The model under review builds one solid part; all positions refer to its coordinate system, in mm. Face numbers are marked on the shaded views. A direction names the side the tool comes from. Round coordinates to 2 decimals unless told otherwise and drop trailing zeros. Order: outer loops, then holes, each group sorted by start corner. A loop starts at its lowest first (then second) coordinate and runs counter-clockwise, first axis right, second up.
1) Machinability: for the marked faces 1, 2, 3 and 4, which of the approach directions +Z, -Z, +X, -X, +Y, -Y give a long, thin tool a straight path to every point of the face, cutting with its end or side? Answer none if there is none.
2) Consider section A-A (y = -14.5). Give the boundary of the cut face in (x, z), then the cut area to 3 significant figures.
3) Consider section B-B (y = -29.5). Give the boundary of the cut face in (x, z), then the cut area to 3 significant figures.
4) Clearance check with flat-ended pins moving along their axes: P1, Ø1.5, axis at y = -12, z = 23.5, coming from the -X side; P2, Ø1.5, axis at x = -19, z = -19.5, coming from the -Y side; P3, Ø4, axis at x = -18.5, y = -9, coming from the +Z side; P4, Ø5, axis at x = -37, z = 37, coming from the -Y side. State where each tip first meets the part, or that it passes through.
5) Mouldability with a two-part tool opening along Z and no side actions: class the marked faces 5, 6 and 7 as pulls with the +Z half, pulls with the -Z half, needs draft (parallel to the pull), parting line crosses it, or undercut.
6) To check wall thickness, follow L1, parallel to Z at x = 37, y = -1; L2, parallel to Z at x = 0, y = -4.35; L3, parallel to Y at x = -34.5, z = -31.5. State the ranges of each line that lie inside material, in increasing order.
from build123d import *

# Parameters (mm, degrees)
F2_W     = 85
F2_H     = 85
F2_R     = 2.75
F3_DEPTH = 5
F4_SIZE  = 1.5
F5_R     = 15
F6_DEPTH = 2


with BuildPart() as f1:
    # F0 (on Right) → F1 (revolve)
    with BuildSketch(Plane.YZ):
        Polygon((-5, 0), (0, 0), (0, 42.5), (-32, 42.5), (-32, 37.7), (-17, 37.7), (-17, 21.2), (-5, 21.2), align=None)
    revolve(axis=Axis((0, -2.5, 0), (0, 1, 0)))

    # F2 (on Front) → F3 (join)
    with BuildSketch(Plane.XZ):
        Rectangle(F2_W, F2_H)
        with Locations((-37, -37)):
            Circle(F2_R, mode=Mode.SUBTRACT)
        with Locations((37, -37)):
            Circle(F2_R, mode=Mode.SUBTRACT)
        with Locations((-37, 37)):
            Circle(F2_R, mode=Mode.SUBTRACT)
        with Locations((37, 37)):
            Circle(F2_R, mode=Mode.SUBTRACT)
    extrude(amount=F3_DEPTH)

    # F4
    f4_edges = [f1.edges().sort_by_distance(p)[0] for p in [
        (0, -32, -37.7),
        (0, -17, -21.2),
        (42.5, -2.5, 42.5),
        (-42.5, -2.5, 42.5),
        (-42.5, -2.5, -42.5),
        (42.5, -2.5, -42.5),
    ]]
    chamfer(f4_edges, length=F4_SIZE)

    # F5 (on face) → F6 (cut)
    with BuildSketch(Plane.XZ.offset(5)):
        Circle(F5_R)
    extrude(amount=-F6_DEPTH, mode=Mode.SUBTRACT)


solid = f1.part
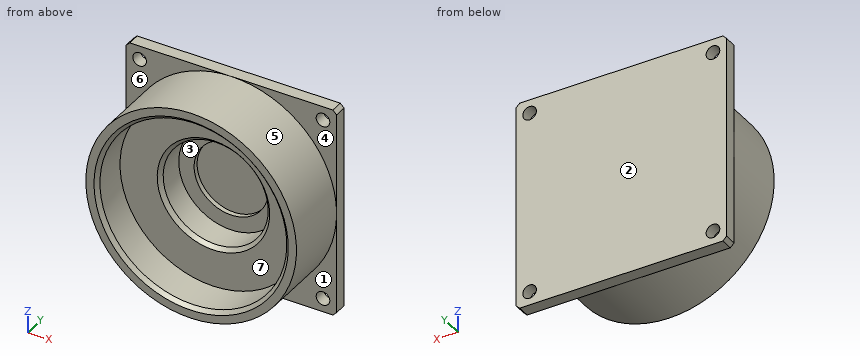
Answer below:
1. face 1: -Z, +X, -Y
1. face 2: +Z, -Z, +X, -X, +Y
1. face 3: -Y
1. face 4: +Z, +X, -Y
2. outline: circle Ø85 at (0, 0); hole circle Ø42.4 at (0, 0)
2. area: 4,260 mm2
3. outline: circle Ø85 at (0, 0); hole circle Ø75.4 at (0, 0)
3. area: 1,210 mm2
4. P1: stops at x = -35.9
4. P2: stops at y = -17
4. P3: stops at z = 39.17
4. P4: passes through
5. face 5: parting line crosses it
5. face 6: needs draft
5. face 7: undercut
6. L1: z = -42.5 to -39.75, -34.25 to 34.25, 39.75 to 42.5
6. L2: z = -42.5 to -15, 15 to 42.5
6. L3: y = -5 to 0
